Geometry: see drawing. Coordinates: mm, zero at the bounding-box minimum. Coordinates: 2 decimals unless noted, no trailing zeros. Write each loop counter-clockwise with the first axis right and the second up, starting at its lowest first coordinate (ties: lowest second). Pieces come first, ordered by that corner, then holes. Notation, with made-up numbers: (-6.5, 42) -> (25.5, 42) arc R31 ccw to (25.5, 66) -> close; hole circle Ø2 at (-24, 26). An arc over 180 degrees is marked (long way). Answer as a JSON object with one key per item and string values. Group by question number.
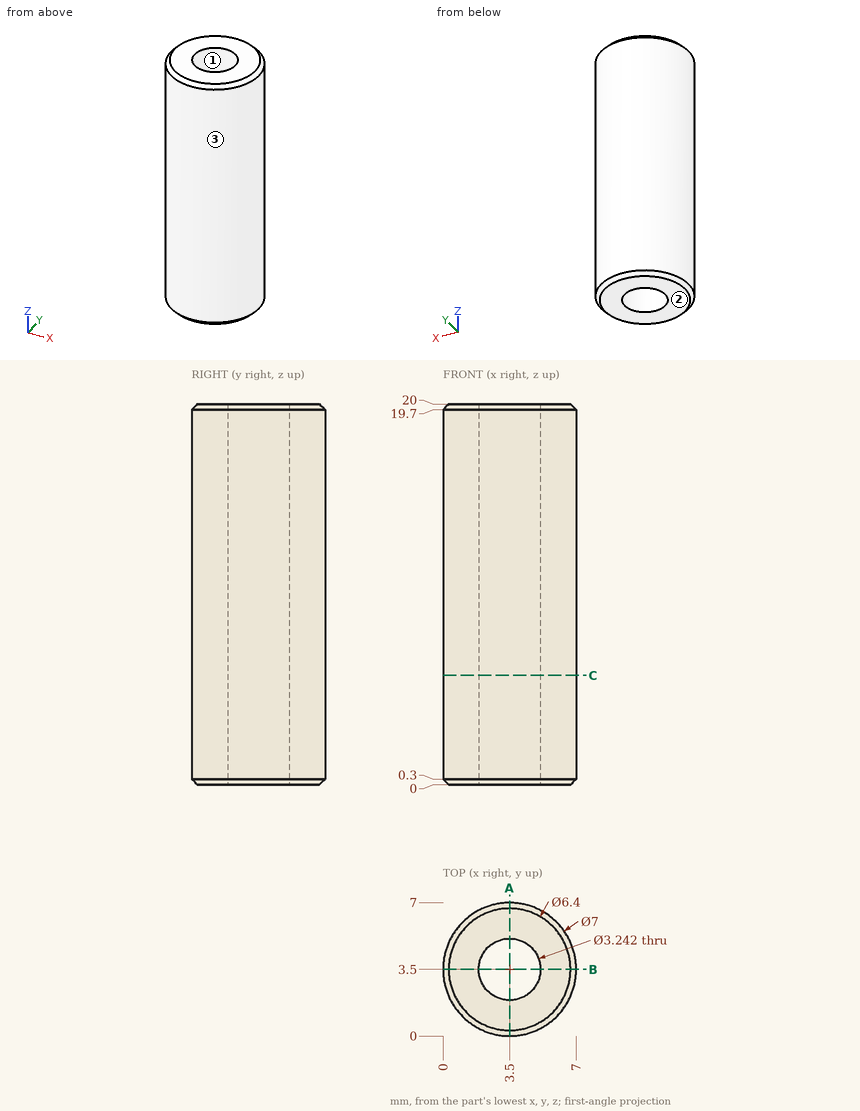
Item 1: Section A-A on x = 3.5. Output: boundary loops of the cut face in (y, z).
Item 2: Ray query, L1, parallel to Y at x = 3.5, z = 6.75; L2, parallel to Z at x = 1, y = 5.5; L3, parallel to Y at x = 3, z = 17.75. Return the intervals inside material, ascending. Write a range as [from, to].
Item 3: Mould query, pull axis Y, two halves, no side actions, for the marked faces 1, 2 and 3. Classes: +Y half, -Y half, draft (parallel to the pull), parting line (faces both ways), or undercut.
Item 4: Section C-C on z = 5.75. Output: boundary loops of the cut face in (x, y).
Answer sheet:
{
 "1": {"outline": "(0, 0.3) -> (0.3, 0) -> (1.88, 0) -> (1.88, 20) -> (0.3, 20) -> (0, 19.7) -> close; (5.12, 0) -> (6.7, 0) -> (7, 0.3) -> (7, 19.7) -> (6.7, 20) -> (5.12, 20) -> close"},
 "2": {"L1": "y = [0, 1.88], [5.12, 7]", "L2": "z = [0, 20]", "L3": "y = [0.04, 1.96], [5.04, 6.96]"},
 "3": {"face 1": "undercut", "face 2": "draft", "face 3": "parting line"},
 "4": {"outline": "circle Ø7 at (3.5, 3.5); hole circle Ø3.24 at (3.5, 3.5)"}
}
